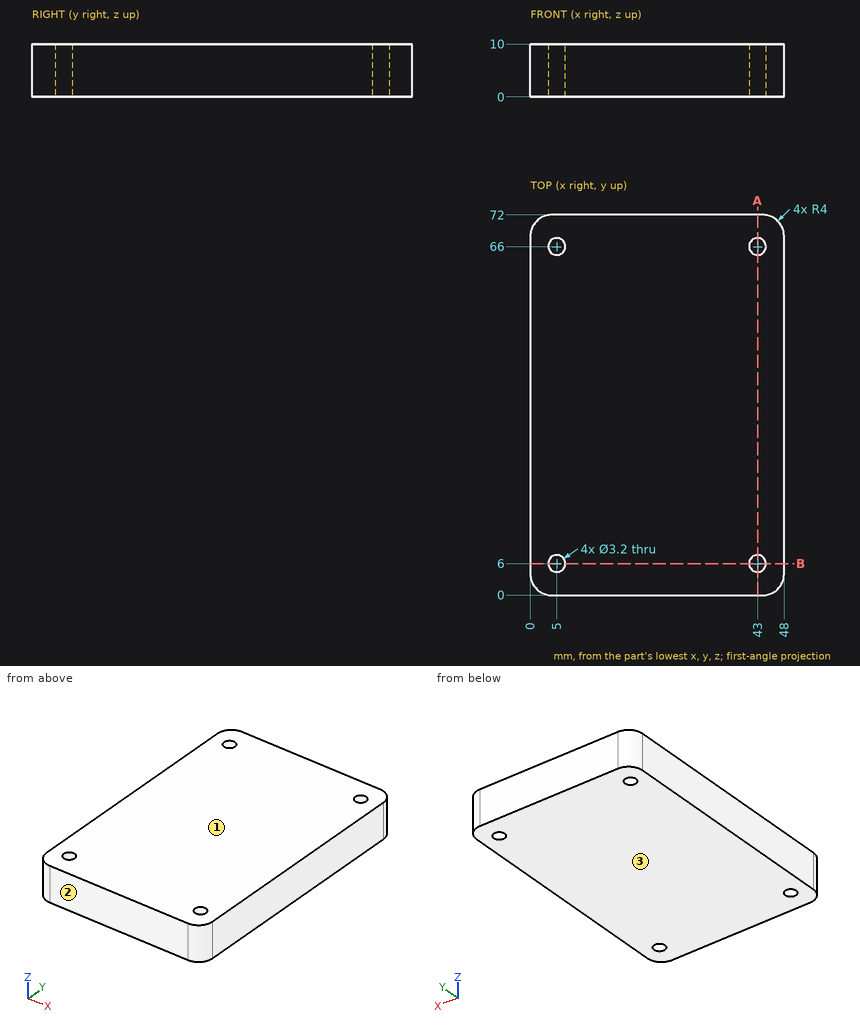
Source: three-view drawing plus pictorial views. Frame: mm from the lowest corner of the part. Give positions to 0.01 mm unless a question says otherwise; leave off trailing zeros. Order: outer loops, then holes, each group sorted by start corner. A loop starts at its lowest first (then second) coordinate and runs counter-clockwise, first axis right, second up. Notation, with made-up numbers: M 88,50 L 110,50 A22 cw 110,67 Z; hole C 16.25,80.5 d11. An arc over 180 degrees is marked long. Return JSON: item names as keys, results as strings.
Item 1: Cut plane A-A (x = 43). Return loops of the section in (y, z).
Solutions:
{"outline": "M 0,0 L 4.4,0 L 4.4,10 L 0,10 Z; M 7.6,0 L 64.4,0 L 64.4,10 L 7.6,10 Z; M 67.6,0 L 72,0 L 72,10 L 67.6,10 Z"}
Item 2: Ray query, probe 1 along Y at (x, z) = (5, 5.5); probe 2 along X at (y, z) = (66, 3); probe 3 along Y at (x, z) = (6, 7.5). Return the intervals inside material, ascending.
Solutions:
{"probe 1": "0 to 4.4, 7.6 to 64.4, 67.6 to 72", "probe 2": "0 to 3.4, 6.6 to 41.4, 44.6 to 48", "probe 3": "0 to 4.75, 7.25 to 64.75, 67.25 to 72"}
Item 3: First-contact query: P1, Ø2.5, axis at x = 43, y = 6, coming from the -Z side. Flat tip, straight axial feed; report the tip coordinate or a pass-through.
Solutions:
{"P1": "through"}
Item 4: Cut plane B-B (y = 6). Return loops of the section in (x, z), then the cut area to 3 significant figures.
Solutions:
{"outline": "M 0,0 L 3.4,0 L 3.4,10 L 0,10 Z; M 6.6,0 L 41.4,0 L 41.4,10 L 6.6,10 Z; M 44.6,0 L 48,0 L 48,10 L 44.6,10 Z", "area": "416 mm^2"}
Item 5: Pull-direction query (Z, two-part tool) for the marked faces 1, 2 and 3; classes: +Z half, -Z half, draft (parallel to the pull), parting line (faces both ways), or undercut.
Solutions:
{"face 1": "+Z half", "face 2": "draft", "face 3": "-Z half"}
